Can you work these out from the model? Positions are in its coordinate system, mm. Face numbers are marked on the shaded views. A direction names the side the tool comes from. Round coordinates to 2 decimals unless told otherwise and drop trailing zeros. Order: outer loops, then holes, each group sorted by start corner. A loop starts at its lowest first (then second) coordinate and runs counter-clockwise, first axis right, second up.
Q1. For the marked faces 1 and 2, which set-ups out of +Z, -Z, +X, -X, +Y, -Y let a thin tool reach every point of the face, with its end or its side?
Q2. If we section it at B-B (z = 15.5): Please give me the cut outline in (x, y).
Q3. If I drill on line 1 (Z direction, x = 22.5, y = 5.5); line 2 (Z direction, x = 4.5, y = 26); line 3 (X direction, y = 12.5, z = -49.5), over which ranges is the centre line in solid material (lowest first)?
Q4. If we section it at C-C (x = -23): Please give me the cut outline in (y, z), plus the area to 3 significant figures.
Q5. We'd pull the mould along X, two halves only. Please class the marked faces 3, 4, 5 and 6: pulls with the +X half, pulls with the -X half, needs draft (parallel to the pull), parting line crosses it, or undercut.
Q6. Will these pins go through, and if not, where does the flat tip stop? P1, Ø0.7, axis at x = 3.5, z = -36, coming from the +Y side; P2, Ø4, axis at y = 17, z = -84, coming from the -X side; P3, Ø1, axis at x = -10, y = 3.5, coming from the -Z side.
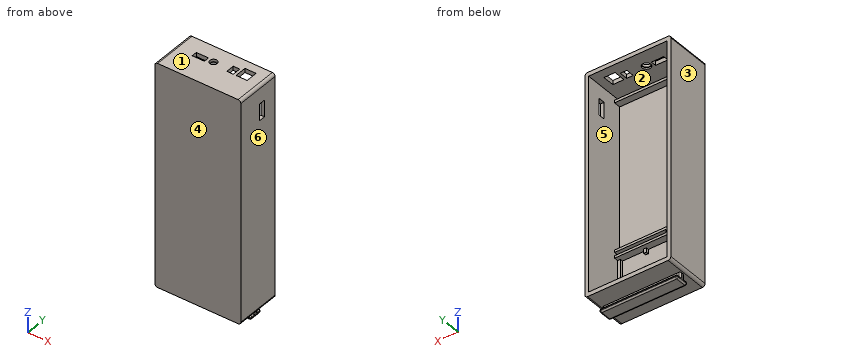
Autodesk Inventor part; units mm, degrees
ref_plane "YZ Plane" through (0, 0, 0) normal (1, 0, 0) x (0, 1, 0)
ref_plane "XZ Plane" through (0, 0, 0) normal (0, 1, 0) x (-1, 0, 0)
ref_plane "XY Plane" through (0, 0, 0) normal (0, 0, 1) x (1, 0, 0)
sketch "Sketch1" plane through (0, 0, 0) normal (0, 1, 0) x (-1, 0, 0)
  line L0 (-31.2, -81) -> (31.2, -81)
  line L1 (31.2, -81) -> (31.2, 81)
  line L2 (31.2, 81) -> (-31.2, 81)
  line L3 (-31.2, 81) -> (-31.2, -81)
  line L4 (-31.2, -81) -> (31.2, 81) construction
  line L5 (31.2, -81) -> (-31.2, 81) construction
  point P0 (0, 0)
  dimension "d0" = 62.4
  dimension "d1" = 162
extrude "Extrusion1" add sketch "Sketch1" along normal blind 3
sketch "Sketch2" plane through (0, 3, 0) normal (0, 1, 0) x (1, 0, 0)
  line L0 (-31.2, 81) -> (-31.2, -81)
  line L1 (-31.2, -81) -> (31.2, -81)
  line L2 (31.2, -81) -> (31.2, 81)
  line L3 (31.2, 81) -> (-31.2, 81)
  line L4 (31.2, 81) -> (-31.2, 81)
  line L5 (-31.2, 81) -> (-31.2, -81)
  line L6 (-31.2, -81) -> (31.2, -81)
  line L7 (31.2, -81) -> (31.2, 81)
  line L8 (28.5, 78) -> (-28.5, 78)
  line L9 (-28.5, 78) -> (-28.5, -78)
  line L10 (-28.5, -78) -> (28.5, -78)
  line L11 (28.5, -78) -> (28.5, 78)
  point P0 (0, 0)
  dimension "d175" = 2.7
  dimension "d176" = 2.7
  dimension "d177" = 3
  dimension "d178" = 3
extrude "Extrusion2" add sketch "Sketch2" along normal blind 30
fillet "Fillet1" radius 2 4 edges at (31.2, 16.5, 81) (31.2, 16.5, -81) (-31.2, 16.5, 81) (-31.2, 16.5, -81)
sketch "Sketch9" plane through (0, 3, 0) normal (0, 1, 0) x (1, 0, 0)
  line L0 (28.5, 78) -> (-28.5, 78)
  line L1 (-28.5, 78) -> (-28.5, -78)
  line L2 (-28.5, -78) -> (28.5, -78)
  line L3 (28.5, -78) -> (28.5, 78)
  line L4 (-28.5, -75.5) -> (28.5, -75.5)
  line L5 (28.5, -75.5) -> (28.5, -73.6)
  line L6 (28.5, -73.6) -> (-28.5, -73.6)
  line L7 (-28.5, -73.6) -> (-28.5, -75.5)
  line L8 (-28.5, 78) -> (-28.5, -78)
  line L9 (-28.5, 32.8) -> (28.5, 32.8)
  line L10 (28.5, 32.8) -> (28.5, 34.55)
  line L11 (28.5, 34.55) -> (-28.5, 34.55)
  line L12 (-28.5, 34.55) -> (-28.5, 32.8)
  line L13 (-28.5, 34.55) -> (-11.1, 34.55)
  line L14 (-11.1, 34.55) -> (-11.1, 32.8)
  line L15 (-11.1, 32.8) -> (-28.5, 32.8)
  line L16 (-28.5, 32.8) -> (-28.5, 34.55)
  line L17 (28.5, 38.7) -> (-11.1, 38.7)
  line L18 (-11.1, 38.7) -> (-11.1, 36.95)
  line L19 (-11.1, 36.95) -> (28.5, 36.95)
  line L20 (28.5, 36.95) -> (28.5, 38.7)
  line L21 (-11.1, 36.95) -> (-8.7, 36.95)
  line L22 (-8.7, 36.95) -> (-8.7, 34.55)
  line L23 (-8.7, 34.55) -> (-11.1, 34.55)
  line L24 (-11.1, 34.55) -> (-11.1, 36.95)
  point P0 (0, 0)
  point P1 (28.5, 14.2)
  point P2 (-28.5, 34.55)
  point P3 (-28.5, 32.8)
  point P4 (28.5, 32.8)
  point P5 (-28.5, -73.6)
  point P6 (28.5, -75.5)
  point P7 (-11.1, 34.55)
  point P8 (28.5, 36.95)
  dimension "d79" = 1.9
  dimension "d80" = 2.5
  dimension "d81" = 1.75
  dimension "d82" = 106.4
  dimension "d87" = 17.4
  dimension "d163" = 1.75
  dimension "d164" = 2.4
  dimension "d165" = 17.4
  dimension "d166" = 2.4
extrude "Extrusion9" add sketch "Sketch9" along normal blind 5 contours L3 L19 L18 L17 | L24 L19 L22 L11 | L11 L3 L9 L14 | L6 L3 L4 L1
sketch "Sketch10" plane through (0, 3, 0) normal (0, 1, 0) x (1, 0, 0)
  line L0 (-28.5, -73.6) -> (28.5, -73.6)
  line L1 (28.5, -73.6) -> (28.5, 32.8)
  line L2 (28.5, 32.8) -> (-11.1, 32.8)
  line L3 (-8.7, 34.55) -> (28.5, 34.55)
  line L4 (28.5, 34.55) -> (28.5, 36.95)
  line L5 (28.5, 78) -> (-28.5, 78)
  line L6 (-28.5, 78) -> (-28.5, -73.6)
  line L7 (-28.5, 36.7) -> (28.5, 36.7)
  line L8 (-28.5, 69.9) -> (-28.5, 36.7)
  line L9 (-28.5, 36.7) -> (28.5, 36.7)
  line L10 (28.5, 36.7) -> (28.5, 38.7)
  line L11 (28.5, 38.7) -> (-28.5, 38.7)
  line L12 (-28.5, 38.7) -> (-28.5, 36.7)
  line L13 (28.5, 34.55) -> (28.5, 78)
  line L14 (-28.5, 38.7) -> (28.5, 38.7)
  line L15 (28.5, 38.7) -> (28.5, 75.6)
  line L16 (28.5, 75.6) -> (-23, 75.6)
  line L17 (-23, 75.6) -> (28.5, 75.6)
  line L18 (28.5, 75.6) -> (28.5, 68)
  line L19 (-23, 73.1) -> (-23, 75.6)
  line L20 (28.5, 38.7) -> (26.5, 38.7)
  line L21 (26.5, 38.7) -> (26.5, 75.6)
  line L22 (26.5, 75.6) -> (28.5, 75.6)
  line L23 (28.5, 75.6) -> (28.5, 38.7)
  line L24 (26.5, 38.7) -> (9.7, 38.7)
  line L25 (9.7, 38.7) -> (9.7, 75.6)
  line L26 (9.7, 75.6) -> (26.5, 75.6)
  line L27 (26.5, 75.6) -> (26.5, 38.7)
  line L28 (9.7, 38.7) -> (7.7, 38.7)
  line L29 (7.7, 38.7) -> (7.7, 75.6)
  line L30 (7.7, 75.6) -> (9.7, 75.6)
  line L31 (9.7, 75.6) -> (9.7, 38.7)
  line L32 (7.7, 38.7) -> (-9.1, 38.7)
  line L33 (-9.1, 38.7) -> (-9.1, 75.6)
  line L34 (-9.1, 75.6) -> (7.7, 75.6)
  line L35 (7.7, 75.6) -> (7.7, 38.7)
  line L36 (-9.1, 38.7) -> (-11.1, 38.7)
  line L37 (-11.1, 38.7) -> (-11.1, 75.6)
  line L38 (-11.1, 75.6) -> (-9.1, 75.6)
  line L39 (-9.1, 75.6) -> (-9.1, 38.7)
  line L40 (-23, 75.6) -> (-21.5, 75.6)
  line L41 (-21.5, 75.6) -> (-21.5, 38.7)
  line L42 (-21.5, 38.7) -> (-23, 38.7)
  line L43 (-23, 38.7) -> (-23, 75.6)
  line L44 (-11.1, 39.2) -> (-11.1, 57)
  line L45 (-11.1, 57) -> (-21.5, 57)
  line L46 (-21.5, 57) -> (-21.5, 38.7)
  line L47 (-11.1, 38.7) -> (28.5, 38.7)
  line L48 (28.5, 38.7) -> (28.5, 78)
  line L49 (-11.1, 32.8) -> (-11.1, 38.7)
  line L50 (28.5, 36.95) -> (-8.7, 36.95)
  line L51 (-8.7, 36.95) -> (-8.7, 34.55)
  line L52 (28.5, -75.5) -> (-28.5, -75.5)
  line L53 (-28.5, -75.5) -> (-28.5, -78)
  line L54 (-28.5, -78) -> (28.5, -78)
  line L55 (28.5, -78) -> (28.5, -75.5)
  line L56 (-11.1, 39.2) -> (-11.1, 36.7)
  line L57 (-11.1, 55) -> (-23, 55)
  line L58 (-11.1, 39.2) -> (-11.1, 32.8)
  line L59 (-11.1, 32.8) -> (-11.1, 32.8)
  line L60 (-11.1, 32.8) -> (-11.1, 39.2)
  line L61 (-23, 55) -> (-28.5, 55)
  line L62 (7.7, 51.8) -> (9.7, 51.8)
  line L63 (9.7, 51.8) -> (9.7, 41.8)
  line L64 (9.7, 41.8) -> (7.7, 41.8)
  line L65 (7.7, 41.8) -> (7.7, 51.8)
  line L66 (-11.1, 41.8) -> (-9.1, 41.8)
  line L67 (-9.1, 41.8) -> (-9.1, 51.8)
  line L68 (-9.1, 51.8) -> (-11.1, 51.8)
  line L69 (-11.1, 51.8) -> (-11.1, 41.8)
  line L70 (-11.1, 71.3) -> (-9.1, 71.3)
  line L71 (-9.1, 71.3) -> (-9.1, 61.3)
  line L72 (-9.1, 61.3) -> (-11.1, 61.3)
  line L73 (-11.1, 61.3) -> (-11.1, 71.3)
  point P0 (0, 0)
  point P1 (28.5, 36.7)
  point P2 (7.7, 38.7)
  point P3 (-9.1, 38.7)
  point P4 (-11.1, 38.7)
  point P5 (-21.5, 38.7)
  point P6 (-21.5, 57)
  point P7 (26.5, 38.7)
  point P8 (9.7, 38.7)
  point P9 (28.2, 37.2)
  point P10 (-11.1, 36.7)
  point P11 (-25.2, 72.6)
  point P12 (-11.1, 75.6)
  point P13 (-11.1, 36.7)
  point P14 (-11.1, 38.7)
  point P15 (-21.5, 75.6)
  point P16 (-25.2, 52)
  point P17 (-11.1, 36.7)
  point P18 (-28.5, 38.7)
  point P19 (28.5, 75.6)
  point P20 (28.5, 38.7)
  point P21 (-11.1, 36.7)
  point P22 (-11.1, 38.7)
  point P23 (-21.5, 55)
  point P24 (-11.1, 38.7)
  point P25 (-10.7, 32.8)
  point P26 (28.5, 38.7)
  point P27 (-11.1, 38.7)
  point P28 (-9.1, 38.7)
  point P29 (-28.5, 55)
  point P30 (7.7, 41.8)
  point P31 (-9.1, 41.8)
  point P32 (-9.1, 51.8)
  point P33 (-11.1, 61.3)
  point P34 (7.7, 51.8)
  point P35 (9.7, 51.8)
  dimension "d90" = 2
  dimension "d91" = 36.9
  dimension "d93" = 2
  dimension "d94" = 16.8
  dimension "d95" = 2
  dimension "d96" = 16.8
  dimension "d97" = 2
  dimension "d98" = 1.5
  dimension "d167" = 2.4
  dimension "d172" = 18.6
  dimension "d173" = 2
  dimension "d174" = 10.4
  dimension "d179" = 10
  dimension "d180" = 10
  dimension "d181" = 3.1
  dimension "d182" = 3.1
  dimension "d183" = 10
  dimension "d184" = 4.3
extrude "Extrusion10" add sketch "Sketch10" along normal blind 2 contours L6 L5 L13 L16 L19 L43 L61 | L37 L66 L33 L11 | L43 L19 L16 L41 L57 | L41 L45 L37 L57 | L29 L64 L25 L11 | L37 L72 L33 L68 | L11 L21 L16 L13 | L29 L16 L25 L62 | L16 L33 L70 L37
sketch "Sketch11" plane through (-23.2, 5, 81) normal (0, 0, 1) x (1, 0, 0)
  line L0 (-6, 28) -> (52.4, 28)
  line L1 (5.5, 13) -> (14.4, 13)
  line L2 (14.4, 13) -> (14.4, 17)
  line L3 (14.4, 17) -> (5.5, 17)
  line L4 (5.5, 17) -> (5.5, 13)
  line L5 (45.4, 13) -> (37.34, 13)
  line L6 (37.34, 13) -> (37.34, 21.6)
  line L7 (37.34, 21.6) -> (45.4, 21.6)
  line L8 (45.4, 21.6) -> (45.4, 13)
  circle A0 centre (19, 15.65) radius 2.65
  line L9 (48.4, 0) -> (48.4, 30)
  line L10 (52.4, 28) -> (52.4, -5)
  line L11 (-6, -5) -> (-6, 28)
  line L12 (-6, -5) -> (52.4, -5)
  line L13 (54.4, -5) -> (54.4, 28)
  line L14 (-8, 28) -> (-8, -5)
  line L15 (30.64, 13) -> (35.34, 13)
  line L16 (35.34, 13) -> (35.34, 19.2)
  line L17 (35.34, 19.2) -> (30.64, 19.2)
  line L18 (30.64, 19.2) -> (30.64, 13)
  point P0 (23.2, -5)
  point P1 (46.4, 0)
  point P2 (0, 0)
  dimension "d110" = 8.9
  dimension "d111" = 4
  dimension "d112" = 8.06
  dimension "d113" = 8.6
  dimension "d114" = 5.3
  dimension "d149" = 9
  dimension "d150" = 13.5
  dimension "d151" = 27
  dimension "d152" = 18
  dimension "d153" = 18
  dimension "d154" = 18
  dimension "d168" = 4.7
  dimension "d169" = 6.2
  dimension "d170" = 2
  dimension "d171" = 18
extrude "Extrusion11" cut sketch "Sketch11" against normal blind 3 contours L4 L3 L2 L1 | L5 L6 L7 L8 | A0 | L18 L17 L16 L15
sketch "Sketch12" plane through (28.5, 3, 78) normal (0, 0, -1) x (-1, 0, 0)
  line L0 (14.36, 23.6) -> (14.36, 15)
  line L1 (14.36, 15) -> (6.3, 15)
  line L2 (6.3, 15) -> (6.3, 23.6)
  line L3 (6.3, 23.6) -> (14.36, 23.6)
  line L4 (37.3, 19) -> (46.2, 19)
  line L5 (46.2, 19) -> (46.2, 15)
  line L6 (46.2, 15) -> (37.3, 15)
  line L7 (37.3, 15) -> (37.3, 19)
  circle A0 centre (32.7, 17.65) radius 2.65
  line L8 (57, 0) -> (0, 0)
  line L9 (57, 0) -> (57, 30)
  line L10 (0, 30) -> (57, 30)
  line L11 (0, 0) -> (0, 30)
  circle A1 centre (32.7, 17.65) radius 3.1
  point P0 (28.5, -3)
  dimension "d128" = 6.2
extrude "Extrusion12" cut sketch "Sketch12" against normal blind 1.2 contours A1
sketch "Sketch13" plane through (23.2, 5, -81) normal (0, 0, -1) x (-1, 0, 0)
  line L0 (-5, 18) -> (51.4, 18)
  line L1 (51.4, 18) -> (51.4, 8.4)
  line L2 (51.4, 8.4) -> (-5, 8.4)
  line L3 (-5, 8.4) -> (-5, 18)
  line L4 (54.4, -5) -> (54.4, 28)
  line L5 (-8, 28) -> (-8, -5)
  line L6 (-6, -5) -> (52.4, -5)
  point P0 (23.2, -5)
  point P1 (51.4, 0)
  point P2 (-5, 0)
  point P3 (54.4, 11.5)
  point P4 (51.4, 13.2)
  dimension "d131" = 9.6
  dimension "d146" = 3
  dimension "d147" = 3
  dimension "d156" = 23
extrude "Extrusion13" add sketch "Sketch13" along normal blind 6
sketch "Sketch14" plane through (-28.2, 13.4, -81) normal (-1, 0, 0) x (0, 0, 1)
  line L0 (0, 9.6) -> (0, 0)
  line L1 (0, 9.6) -> (-6, 9.6)
  line L2 (-6, 0) -> (-6, 9.6)
  line L3 (0, 0) -> (-6, 0)
  line L4 (0, 9.6) -> (-3.4, 9.6)
  line L5 (-3.4, 9.6) -> (-3.4, 6.6)
  line L6 (-3.4, 6.6) -> (0, 6.6)
  line L7 (0, 6.6) -> (0, 9.6)
  line L8 (0, 0) -> (-3.4, 0)
  line L9 (-3.4, 0) -> (-3.4, 3)
  line L10 (-3.4, 3) -> (0, 3)
  line L11 (0, 3) -> (0, 0)
  point P0 (81, -13.4)
  point P1 (0, 6.6)
  dimension "d137" = 3.4
  dimension "d138" = 3
  dimension "d139" = 3.4
  dimension "d140" = 3
extrude "Extrusion14" cut sketch "Sketch14" against normal up to surface (56.4 mm away) contours L0 L6 L5 L1 | L0 L3 L9 L10
fillet "Fillet5" radius 1 18 edges at (0, 23, -87) (0, 23, -84.4) (0, 13.4, -87) (0, 13.4, -84.4) (-28.2, 16.4, -82.7) (-28.2, 20, -82.7) (28.2, 16.4, -82.7) (28.2, 20, -82.7) (-28.2, 18.2, -87) (-28.2, 21.5, -84.4) (-28.2, 14.9, -84.4) (-28.2, 23, -85.7) (-28.2, 13.4, -85.7) (28.2, 23, -85.7) (28.2, 13.4, -85.7) (28.2, 14.9, -84.4) (28.2, 18.2, -87) (28.2, 21.5, -84.4)
sketch "Sketch15" plane through (31.2, 0, 79) normal (1, 0, 0) x (0, 0, -1)
  line L0 (11, 22.8) -> (23.1, 22.8)
  line L1 (23.1, 22.8) -> (23.1, 18)
  line L2 (23.1, 18) -> (11, 18)
  line L3 (11, 18) -> (11, 22.8)
  line L4 (-2, 33) -> (-2, 0)
  line L5 (0, 0) -> (158, 0)
  point P0 (79, 0)
  dimension "d157" = 12.1
  dimension "d158" = 4.8
  dimension "d159" = 13
  dimension "d160" = 18
extrude "Extrusion15" cut sketch "Sketch15" against normal blind 3
properties part number "module_command" material "PC/ABS Plastic"
Solution:
1. face 1: +Z, +X, -X, +Y, -Y
1. face 2: +Y
2. outline: (-31.2, 0) - (31.2, 0) - (31.2, 33) - (28.5, 33) - (28.5, 3) - (-28.5, 3) - (-28.5, 33) - (-31.2, 33) - close
3. line 1: z = -81 to -78, -38.7 to -36.95, -34.55 to -32.8, 73.6 to 75.5, 78 to 81
3. line 2: z = -81 to -78, 78 to 81
3. line 3: x = -31.2 to -28.5, 28.5 to 31.2
4. outline: (0, -81) - (16.4, -81) - (16.4, -84.4) - (14.4, -84.4) arc R1 ccw to (13.4, -85.4) - (13.4, -86) arc R1 ccw to (14.4, -87) - (22, -87) arc R1 ccw to (23, -86) - (23, -85.4) arc R1 ccw to (22, -84.4) - (20, -84.4) - (20, -81) - (33, -81) - (33, -78) - (5, -78) - (5, -55) - (3, -55) - (3, 73.6) - (8, 73.6) - (8, 75.5) - (3, 75.5) - (3, 78) - (33, 78) - (33, 81) - (0, 81) - close
4. area: 758 mm2
5. face 3: pulls with the -X half
5. face 4: needs draft
5. face 5: undercut
5. face 6: pulls with the +X half
6. P1: stops at y = 3
6. P2: stops at x = -28.2
6. P3: stops at z = -81
